Autodesk Inventor part; units mm, degrees
ref_plane "YZ Plane" through (0, 0, 0) normal (1, 0, 0) x (0, 1, 0)
ref_plane "XZ Plane" through (0, 0, 0) normal (0, 1, 0) x (-1, 0, 0)
ref_plane "XY Plane" through (0, 0, 0) normal (0, 0, 1) x (1, 0, 0)
sketch "Sketch2" plane through (0, 0, 0) normal (1, 0, 0) x (0, 1, 0)
  circle A0 centre (0, 0) radius 10
  circle A1 centre (0, 0) radius 22
  line L0 (0, 0) -> (7.0711, -7.0711)
  line L1 (0, 0) -> (10, 0) construction
  circle A2 centre (7.0711, -7.0711) radius 1.5
  line L2 (0, 0) -> (10.8294, 10.8294)
  line L3 (0, 0) -> (15.315, 0) construction
  circle A3 centre (-7.0711, 7.0711) radius 1.5
  dimension "d3" = 20
  dimension "d4" = 44
  dimension "d16" = 10
  dimension "d17" = 45
  dimension "d18" = 3
  dimension "d19" = 45
extrude "Extrusion1" add sketch "Sketch2" along normal blind 12 contours A2 A0 | A0 L0 A2 | A3 A0 | A0 A3 | A0 A2 L0 | A1
sketch "Sketch4" plane through (0, 0, 0) normal (1, 0, 0) x (0, 0, -1)
  circle A0 centre (0, 0) radius 15.75
  circle A1 centre (15.75, 0) radius 2.55
  dimension "d9" = 31.5
  dimension "d10" = 5.1
extrude "Extrusion3" cut sketch "Sketch4" along normal blind 30 contours A0 A1 | A0 A1 picked at (14.9184, -0.4924) picked at (16.4994, -0.6699)
sketch "Sketch5" plane through (12, 0, 0) normal (1, 0, 0) x (0, 0, -1)
  circle A0 centre (15.75, 0) radius 2.55
  circle A1 centre (15.75, 0) radius 4.5
  point P0 (0, 0)
  dimension "d20" = 9
extrude "Extrusion4" cut sketch "Sketch5" against normal blind 4
sketch "Sketch6" plane through (12, 0, 0) normal (1, 0, 0) x (0, 0, -1)
  line L0 (0, 0) -> (15.5563, 15.5563)
  line L1 (0, 0) -> (22, 0) construction
  dimension "d23" = 22
  dimension "d24" = 45
ref_plane "Work Plane1" through (12, 15.5563, -15.5563) normal (0, 0.7071068, -0.7071068) x (-1, 0, 0)
sketch "Sketch7" plane through (12, 15.5563, -15.5563) normal (0, 0.7071068, -0.7071068) x (-1, 0, 0)
  line L0 (0, 22) -> (0, -22)
  line L1 (0, 0) -> (12, 0)
  circle A0 centre (6, 0) radius 2.6
  dimension "d25" = 5.2
extrude "Extrusion5" cut sketch "Sketch7" against normal blind 10
ref_plane "Work Plane2" through (12, 0, 0) normal (0, 0.7071068, -0.7071068) x (-1, 0, 0)
thread "Thread1"
mirror "Mirror1" about plane through (12, 0, 0) normal (0, 0.7071068, -0.7071068) of "Extrusion5"
sketch "Sketch8" plane through (12, 0, 0) normal (1, 0, 0) x (0, 0, -1)
  line L0 (0, 0) -> (22, 0) construction
  circle A0 centre (15.75, 0) radius 2.55
  circle A1 centre (15.75, 0) radius 5
  dimension "d33" = 10
extrude "Extrusion6" cut sketch "Sketch8" against normal blind 2
chamfer "Chamfer2" distance 0.5 angle 45 1 edges at (10, 0, -11.25)
pattern_circular "Circular Pattern1" count 4 over 360 about axis through (-10, 0, 0) along (1, 0, 0) of "Extrusion3", "Extrusion4", "Extrusion6", "Chamfer2"
properties part number "Pen Holder Interface V2"
Can you work these out from the model? Positions are in its coordinate system, mm. A direction names the side the tool comes from. Round coordinates to 2 decimals unless told otherwise and drop trailing zeros. Write each loop counter-clockwise with the first axis right and the second up, starting at its lowest first coordinate (ties: lowest second). Pieces come first, ordered by that corner, then holes. Notation, with made-up numbers: (-21, 88.25) -> (5, 88.25) arc R5 ccw to (5, 93.25) -> close; hole circle Ø2 at (-0.5, 84). An arc over 180 degrees is marked (long way). Use one line per item in the form item = value. Start each with the question number.
Q1. If I drill on probe 1 along Y at (x, z) = (5.25, 9); probe 2 along Z at (x, y) = (6.25, -1.5); probe 3 along Z at (x, y) = (7.75, 9), over which ranges is the centre line in solid material (lowest first)? Write a range as [from, to].
Q2. Imagine slicing it at A-A (z = 0). Count the separate pieces of the cut face and the enclosed holes in it, then the cut area to 3 significant figures.
Q3. Imagine slicing it at B-B (x = 5). Please give me the cut outline in (y, z), then the cut area to 3 significant figures.
Q4. We'd pull the mould along X, two halves only. Please class faces 3 (the face through (8, -2, -18)), 4 (the face through (3.9, -13.2, 0.1)), 5 (the face through (5.96, -8.46, 8.51)): +X half, -X half, draft (parallel to the pull), parting line (faces both ways), or undercut.
Q5. Which directions (+Z, -Z, +X, -X, +Y, -Y) give clear straight access to the entire face, cutting with the end or side of a thin tool? Please do faces 1 (the face through (12, 9, -5)), 2 (the face through (8.761, 11.254, 0.198)).
Q6. I'm going to push flat-ended pins straight in: P1, Ø3, axis at y = -2.5, z = 14.5, coming from the +X side; P2, Ø1, axis at x = 2, z = 17, coming from the -Y side; P3, Ø5, axis at x = 10, z = 3, coming from the +Y side. Where does each tip first touch, or does it pass through?
Worked out:
q1.probe_1 = [-20.07, -12.52], [-7.97, -4.36], [4.36, 20.07]
q1.probe_2 = [-21.95, -17.81], [-13.69, -9.89], [9.89, 13.69], [17.81, 21.95]
q1.probe_3 = [-20.07, -11.72], [-7.97, -4.36], [4.36, 20.07]
q2.separate_pieces = 4
q2.enclosed_holes = 0
q2.area = 130 mm^2
q3.outline = (-17.16, 13.77) arc R22 ccw to (13.77, -17.16) -> (6.79, -10.18) -> (10.18, -6.79) -> (17.16, -13.77) arc R22 ccw to (-13.77, 17.16) -> (-6.79, 10.18) -> (-10.18, 6.79) -> close; hole circle Ø5.1 at (-15.75, 0); hole (-8.05, 5.93) arc R10 ccw to (5.93, -8.05) arc R1.5 cw to (8.05, -5.93) arc R10 ccw to (-5.93, 8.05) arc R1.5 cw to start; hole circle Ø5.1 at (0, -15.75); hole circle Ø5.1 at (0, 15.75); hole circle Ø5.1 at (15.75, 0)
q3.area = 1,040 mm^2
q4.face_3 = +X half
q4.face_4 = draft
q4.face_5 = undercut
q5.face_1 = +Z, -Z, +X, +Y, -Y
q5.face_2 = +X
q6.P1 = 8
q6.P2 = -14.55
q6.P3 = 21.99
